Here's how the part is built. I have some questions about the finished solid (model axes, mm). A direction names the side the tool comes from. Coordinates: 2 decimals unless noted, no trailing zeros. Write each loop counter-clockwise with the first axis right and the second up, starting at its lowest first coordinate (ties: lowest second). Pieces come first, ordered by that corner, then holes. Notation, with made-up numbers: M 44,-4.5 L 77,-4.5 A22 cw 77,24.5 Z; hole C 79.25,6 d1. An arc over 180 degrees is marked long. Use a Markdown table: item, result.
```python
from build123d import *

# Parameters (mm, degrees)
SKETCH1_W           = 3.6
SKETCH1_H           = 11.4
SKETCH1_H_2         = 3.6
SKETCH1_W_2         = 7.8
SKETCH1_R           = 1.8
BOSS_EXTRUDE1_DEPTH = 3.6
SKETCH1_3_W         = 3.6
SKETCH1_3_H         = 11.4
SKETCH1_3_H_2       = 3.6
SKETCH1_3_W_2       = 7.8
BOSS_EXTRUDE2_DEPTH = 22
SKETCH2_W           = 3.6
SKETCH2_H           = 11.4
SKETCH2_W_2         = 7.8
SKETCH2_H_2         = 3.6
BOSS_EXTRUDE3_DEPTH = 2
SKETCH2_3_W         = 3.6
SKETCH2_3_H         = 3.6
SKETCH2_3_H_2       = 11.4
BOSS_EXTRUDE4_DEPTH = 4


with BuildPart() as part:
    # Sketch1 → Boss-Extrude1 (new body)
    # profile 1 of 6: a face of its own
    with BuildSketch(Plane(origin=(0, 0, 0), x_dir=(0, 0, -1), z_dir=(1, 0, 0))):
        with Locations((5.7, -1.8)):
            Rectangle(SKETCH1_W, SKETCH1_H)
    # profile 2 of 6: a face of its own
    with BuildSketch(Plane(origin=(0, 0, 0), x_dir=(0, 0, -1), z_dir=(1, 0, 0))):
        with Locations((5.7, 5.7)):
            Rectangle(SKETCH1_W, SKETCH1_H_2)
    # profile 3 of 6: a face of its own
    with BuildSketch(Plane(origin=(0, 0, 0), x_dir=(0, 0, -1), z_dir=(1, 0, 0))):
        with Locations((0, 5.7)):
            Rectangle(SKETCH1_W_2, SKETCH1_H_2)
    # profile 4 of 6: a face of its own
    with BuildSketch(Plane(origin=(0, 0, 0), x_dir=(0, 0, -1), z_dir=(1, 0, 0))):
        with Locations((-5.7, 5.7)):
            Rectangle(SKETCH1_W, SKETCH1_H_2)
    # profile 5 of 6: a face of its own
    with BuildSketch(Plane(origin=(0, 0, 0), x_dir=(0, 0, -1), z_dir=(1, 0, 0))):
        with Locations((-5.7, -1.8)):
            Rectangle(SKETCH1_W, SKETCH1_H)
    # profile 6 of 6: a face of its own
    with BuildSketch(Plane(origin=(0, 0, 0), x_dir=(0, 0, -1), z_dir=(1, 0, 0))):
        with Locations((0, -1.8)):
            Rectangle(SKETCH1_W_2, SKETCH1_H)
        Circle(SKETCH1_R, mode=Mode.SUBTRACT)
    extrude(amount=-BOSS_EXTRUDE1_DEPTH)

    # Sketch1_3 → Boss-Extrude2 (add)
    with BuildSketch(Plane(origin=(0, 0, 0), x_dir=(0, 0, -1), z_dir=(1, 0, 0))):
        with Locations((-5.7, -1.8)):
            Rectangle(SKETCH1_3_W, SKETCH1_3_H)
        with Locations((-5.7, 5.7)):
            Rectangle(SKETCH1_3_W, SKETCH1_3_H_2)
        with Locations((0, 5.7)):
            Rectangle(SKETCH1_3_W_2, SKETCH1_3_H_2)
        with Locations((5.7, 5.7)):
            Rectangle(SKETCH1_3_W, SKETCH1_3_H_2)
        with Locations((5.7, -1.8)):
            Rectangle(SKETCH1_3_W, SKETCH1_3_H)
    extrude(amount=BOSS_EXTRUDE2_DEPTH)

    # Sketch2 → Boss-Extrude3 (add)
    with BuildSketch(Plane(origin=(22, 0, 0), x_dir=(0, 0, -1), z_dir=(1, 0, 0))):
        with Locations((5.7, -1.8)):
            Rectangle(SKETCH2_W, SKETCH2_H)
        with Locations((0, -1.8)):
            Rectangle(SKETCH2_W_2, SKETCH2_H)
        Polygon((7.5, 7.5), (-3.9, 7.5), (-3.9, 3.9), (3.9, 3.9), (7.5, 3.9), align=None)
        with Locations((-5.7, 5.7)):
            Rectangle(SKETCH2_W, SKETCH2_H_2)
        with Locations((-5.7, -1.8)):
            Rectangle(SKETCH2_W, SKETCH2_H)
    extrude(amount=BOSS_EXTRUDE3_DEPTH)

    # Sketch2_3 → Boss-Extrude4 (add)
    with BuildSketch(Plane(origin=(22, 0, 0), x_dir=(0, 0, -1), z_dir=(1, 0, 0))):
        Polygon((7.5, 7.5), (-3.9, 7.5), (-3.9, 3.9), (3.9, 3.9), (7.5, 3.9), align=None)
        with Locations((-5.7, 5.7)):
            Rectangle(SKETCH2_3_W, SKETCH2_3_H)
        with Locations((-5.7, -1.8)):
            Rectangle(SKETCH2_3_W, SKETCH2_3_H_2)
    extrude(amount=BOSS_EXTRUDE4_DEPTH)


solid = part.part
```
1. Suppose I cut it at A-A on z = 0. Write out the boundary of the cut face in (x, y).
Answers follow:
| item | result |
|---|---|
| outline | M -3.6,-7.5 L 0,-7.5 L 0,-1.8 L -3.6,-1.8 Z; M -3.6,1.8 L 0,1.8 L 0,3.9 L 22,3.9 L 22,-7.5 L 24,-7.5 L 24,3.9 L 26,3.9 L 26,7.5 L -3.6,7.5 Z |
2. We'd pull the mould along Z, two halves only. Please class faces 1 (the face through (0, -2, 1)), 2 (the face through (11, 0, 7.5)), 3 (the face through (25, 3.9, -2)), 4 (the face through (-1.775, 0.541, -1.717)): +Z half, -Z half, draft (parallel to the pull), parting line (faces both ways), or undercut.
Answers follow:
| item | result |
|---|---|
| face 1 | undercut |
| face 2 | +Z half |
| face 3 | draft |
| face 4 | undercut |
3. Suppose I cut it at D-D on y = 0. Write out the boundary of the cut face in (x, z), and give its area (3 significant figures).
Answers follow:
| item | result |
|---|---|
| outline | M -3.6,-7.5 L 24,-7.5 L 24,3.9 L 26,3.9 L 26,7.5 L -3.6,7.5 L -3.6,1.8 L 0,1.8 L 0,3.9 L 22,3.9 L 22,-3.9 L 0,-3.9 L 0,-1.8 L -3.6,-1.8 Z |
| area | 237 mm2 |
4. I need wall thicknesses on probe 1 along X at (y, z) = (-5.5, -1.25); probe 2 along Y at (x, z) = (-1.75, 0); probe 3 along Z at (x, y) = (3.75, -0.75). Which ranges of each line are inside material? Lowest first, please.
Answers follow:
| item | result |
|---|---|
| probe 1 | x = -3.6 to 0, 22 to 24 |
| probe 2 | y = -7.5 to -1.8, 1.8 to 7.5 |
| probe 3 | z = -7.5 to -3.9, 3.9 to 7.5 |
5. Which directions (+Z, -Z, +X, -X, +Y, -Y) give clear straight access to the entire face, cutting with the end or side of a thin tool? Please do faces 5 (the face through (25, -2, 3.9)), 6 (the face through (11, -2, -3.9)), 7 (the face through (26, 5, 3)).
Answers follow:
| item | result |
|---|---|
| face 5 | -Z, +X, -Y |
| face 6 | -Y |
| face 7 | +Z, -Z, +X, +Y, -Y |
6. Will these pins go through, and if not, where does the flat tip stop? pin 1 Ø6 at (y, z) = (-1, -2) entering from +X; pin 2 Ø2.5 at (y, z) = (-0.5, 0) entering from -X; pin 3 Ø2 at (x, y) = (25.5, -1) entering from -Z.
Answers follow:
| item | result |
|---|---|
| pin 1 | stops at x = 24 |
| pin 2 | stops at x = 22 |
| pin 3 | stops at z = 3.9 |
7. Suppose I cut it at C-C on x = -1.5. Write out the boundary of the cut face in (y, z).
Answers follow:
| item | result |
|---|---|
| outline | M -7.5,-7.5 L 7.5,-7.5 L 7.5,7.5 L -7.5,7.5 Z; hole C 0,0 d3.6 |
8. Suppose I cut it at B-B on y = -4.25. Write out the boundary of the cut face in (x, z), and give its area (3 significant figures).
Answers follow:
| item | result |
|---|---|
| outline | M -3.6,-7.5 L 24,-7.5 L 24,3.9 L 26,3.9 L 26,7.5 L -3.6,7.5 Z; hole M 0,-3.9 L 22,-3.9 L 22,3.9 L 0,3.9 Z |
| area | 250 mm2 |
